Input: part model. Units: mm. Frame: model coordinates. Round coordinates to 2 decimals unless told otherwise and drop trailing zeros. Loops run counter-clockwise (first coordinate to the right, second up) from the corner with the lowest first, then second, coordinate; pieces in that order, holes last. Notation, with made-up numbers: (86.25, 63.5) -> (111.25, 63.5) arc R8 ccw to (111.25, 67.5) -> close; hole circle Ø7 at (51, -8.5). An arc over 180 degrees is marked (long way). Answer in a Markdown table with one row per item. Add a question column.
Q1. Section C-C, the plane z = 5. Output: boundary loops of the cut face in (x, y).
Q2. Mould query, pull axis X, two halves, no side actions, for faces 1 (the face through (19, 5, 5)), 2 (the face through (10, 3, 5)), 3 (the face through (20, 2, 5)). Classes: pulls with the +X half, pulls with the -X half, needs draft (parallel to the pull), parting line crosses it, or undercut.
Q3. Ray query, L1, parallel to X at y = 1.2, z = 5; L2, parallel to Z at x = 17, y = 3.3; L3, parallel to X at y = 2.35, z = 6.5. Return the intervals inside material, ascending. Write a range as from..to.
Q4. Section B-B, the plane y = 3.35. Output: boundary loops of the cut face in (x, z).
Q5. Section A-A, the plane x = 17. Output: boundary loops of the cut face in (y, z), and give its area (3 significant figures).
Q6. Pin query (flat end, axial travel): pin 1 (3 mm diameter, centred on x = 17.5, z = 4.5, fed in from +Y). Return the tip coordinate at first contact, or that it passes through.
Q7. Section D-D, the plane z = 9. Output: boundary loops of the cut face in (x, y), and give its area (3 significant figures).
```python
from build123d import *

# Parameters (mm, degrees)
AUFSATZ_LINEAR_AUSTRAGEN1_DEPTH = 10
SKIZZE2_R                       = 1.75
SCHNITT_LINEAR_AUSTRAGEN1_DEPTH = 6


with BuildPart() as part:
    # Skizze1 → Aufsatz-Linear austragen1 (new body)
    with BuildSketch(Plane.XY):
        with BuildLine():
            Line((0, 0), (20, 0))
            Line((20, 0), (20, 5))
            Line((20, 5), (14, 5))
            ThreePointArc((14, 5), (10, 3), (6, 5))
            Line((6, 5), (0, 5))
            Line((0, 5), (0, 0))
        make_face()
    extrude(amount=AUFSATZ_LINEAR_AUSTRAGEN1_DEPTH)

    # Skizze2 → Schnitt-Linear austragen1 (cut, through all)
    with BuildSketch(Plane(origin=(0, 5, 0), x_dir=(1, 0, 0), z_dir=(0, 1, 0))):
        with Locations((3, -5)):
            Circle(SKIZZE2_R)
        with Locations((17, -5)):
            Circle(SKIZZE2_R)
    extrude(amount=-SCHNITT_LINEAR_AUSTRAGEN1_DEPTH, mode=Mode.SUBTRACT)


solid = part.part
```
Answer block:
| question | item | result |
|---|---|---|
| 1 | outline | (0, 0) -> (1.25, 0) -> (1.25, 5) -> (0, 5) -> close; (4.75, 0) -> (15.25, 0) -> (15.25, 5) -> (14, 5) arc R5 cw to (6, 5) -> (4.75, 5) -> close; (18.75, 0) -> (20, 0) -> (20, 5) -> (18.75, 5) -> close |
| 2 | face 1 | needs draft |
| 2 | face 2 | undercut |
| 2 | face 3 | pulls with the +X half |
| 3 | L1 | 0..1.25, 4.75..15.25, 18.75..20 |
| 3 | L2 | 0..3.25, 6.75..10 |
| 3 | L3 | 0..2.1, 3.9..16.1, 17.9..20 |
| 4 | outline | (0, 0) -> (8.16, 0) -> (8.16, 10) -> (0, 10) -> close; (11.84, 0) -> (20, 0) -> (20, 10) -> (11.84, 10) -> close; hole circle Ø3.5 at (3, 5); hole circle Ø3.5 at (17, 5) |
| 5 | outline | (0, 0) -> (5, 0) -> (5, 3.25) -> (0, 3.25) -> close; (0, 6.75) -> (5, 6.75) -> (5, 10) -> (0, 10) -> close |
| 5 | area | 32.5 mm^2 |
| 6 | pin 1 | y = 5 |
| 7 | outline | (0, 0) -> (20, 0) -> (20, 5) -> (14, 5) arc R5 cw to (6, 5) -> (0, 5) -> close |
| 7 | area | 88.8 mm^2 |
